The listing builds one solid part. Answer for the finished solid, in the listing's coordinates (mm). Round coordinates to 2 decimals unless told otherwise and drop trailing zeros. Write each loop counter-clockwise with the first axis right and the second up, starting at its lowest first coordinate (ties: lowest second). Pieces come first, ordered by that corner, then holes.
from build123d import *

# Parameters (mm, degrees)
BOSS_EXTRUDE1_DEPTH         = 3.175
FILLET1_R                   = 3.175
F_1_4_0_25_DIAMETER_HOLE1_D = 6.35


with BuildPart() as part:
    # Sketch1 → Boss-Extrude1 (new body)
    with BuildSketch(Plane(origin=(0, 0, 0), x_dir=(1, 0, 0), z_dir=(0, 1, 0))):
        Polygon((-245.911961207, 0), (245.911961207, 0), (517.525, 708.025), (-517.525, 708.025), align=None)
    extrude(amount=BOSS_EXTRUDE1_DEPTH)

    # Fillet1
    fillet1_edges = [part.edges().sort_by_distance(p)[0] for p in [
        (-517.525, 1.5875, -708.025),
        (517.525, 1.5875, -708.025),
        (245.911961207, 1.5875, 0),
        (-245.911961207, 1.5875, 0),
    ]]
    fillet(fillet1_edges, radius=FILLET1_R)

    # 1/4 (0.25) Diameter Hole1 (through all)
    with Locations(Plane(origin=(0, 3.175, 0), x_dir=(1, 0, 0), z_dir=(0, 1, 0))):
        with Locations((-406.4, 695.325), (0, 695.325), (406.4, 695.325), (-469.681706805, 601.038913991), (-369.60903133, 340.175310506), (-269.536355855, 79.311707021), (269.536355855, 79.311707021), (369.60903133, 340.175310506), (469.681706805, 601.038913991)):
            Hole(F_1_4_0_25_DIAMETER_HOLE1_D / 2)


solid = part.part
1. Section B-B on z = -226.5 is taken. Determine the outline of the cut face in (x, y) (3 decimals), plus the area to 3 significant figures.
Geometry says:
outline: (-332.802, 0) - (332.802, 0) - (332.802, 3.175) - (-332.802, 3.175) - close
area: 2,110 mm2
2. Section C-C on x = 326.5 is taken. Determine the outline of the cut face in (y, z) (3 decimals), plus the area to 3 significant figures.
Geometry says:
outline: (0, -708.025) - (3.175, -708.025) - (3.175, -210.072) - (0, -210.072) - close
area: 1,580 mm2
3. Section A-A on y = 1.7 is taken. Give the number of separate pieces and of enclosed holes in the cut face, plus the area to 3 significant figures.
Geometry says:
separate pieces: 1
enclosed holes: 9
area: 540,000 mm2
4. Straight lines are drawn through the part: line 1 along X through (y, z) = (1.8, -495.5); line 2 along X through (y, z) = (2.85, -399). For each, find the intervals that lie inside material, in ascending order.
Geometry says:
line 1: x = -436 to 436
line 2: x = -398.98 to 398.98
